Read the model definition and answer for the solid it produces. Units are mm, in the model's axes. Face numbers are marked on the shaded views. Coordinates: 2 decimals unless noted, no trailing zeros. Loops run counter-clockwise (first coordinate to the right, second up) from the corner with the lowest first, then second, coordinate; pieces in that order, holes last. Notation, with made-up numbers: (68.5, -24.5) - (102.5, -24.5) arc R11 cw to (102.5, -14.5) - close; hole circle Ø11 at (71.25, 69.25). An arc over 180 degrees is marked (long way). Use one line per item in the form item = value. Start each with the question number.
1) A cutting plane is placed at D-D (z = -13.5). Give the vertices of the cut face in (x, y), and give its area (3 significant figures).
2) The mould has two halves that part along Z. Classify the marked faces 1, 2 and 3: released by +Z, released by -Z, zero draft, split by the parting line, or undercut.
3) A cutting plane is placed at A-A (z = 6). Give the vertices of the cut face in (x, y) (3 decimals).
4) A cutting plane is placed at C-C (x = -11). Give the vertices of the cut face in (y, z).
5) Consider line 1 (Z direction, x = 22, y = 3.6); line 2 (X direction, y = 3.45, z = 14.5); line 3 (X direction, y = 0.85, z = -10). Determine where each line is inside the solid, lowest interval first.
6) This flat-tipped pin is pushed along its axis until it touches: P1, Ø2, axis at x = 21, z = 14.5, coming from the +Y side. Where does it stop, or does it pass through?
7) A cutting plane is placed at B-B (y = 4.3). Give the vertices of the cut face in (x, z).
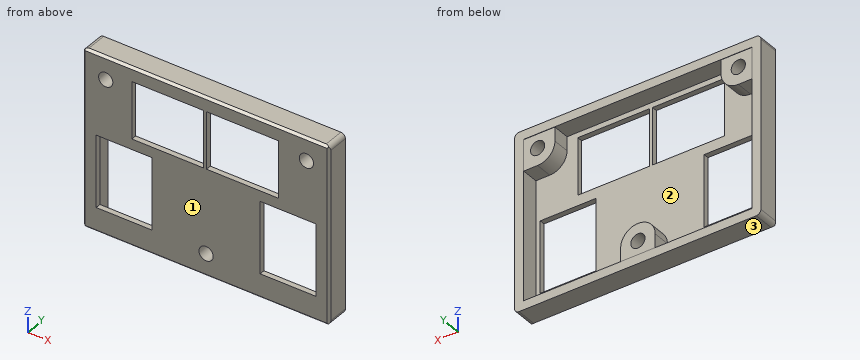
from build123d import *

# Parameters (mm, degrees)
SKETCH1_W           = 54
SKETCH1_H           = 39
BOSS_EXTRUDE1_DEPTH = 5
SKETCH2_W           = 50.1
SKETCH2_H           = 35.1
CUT_EXTRUDE1_DEPTH  = 0.0762
CUT_EXTRUDE2_DEPTH  = 3.75
SKETCH4_R           = 1.56
CUT_EXTRUDE3_DEPTH  = 34.667399758
SKETCH6_W           = 12.25
SKETCH6_H           = 15.75
SKETCH6_W_2         = 15.75
SKETCH6_H_2         = 12.5
CUT_EXTRUDE5_DEPTH  = 34.524465789
CHAMFER1_SIZE       = 0.5
FILLET1_R           = 1


with BuildPart() as part:
    # Sketch1 → Boss-Extrude1 (new body)
    with BuildSketch(Plane(origin=(0, 0, 0), x_dir=(1, 0, 0), z_dir=(0, 1, 0))):
        Rectangle(SKETCH1_W, SKETCH1_H)
    extrude(amount=BOSS_EXTRUDE1_DEPTH)

    # Sketch2 → Cut-Extrude1 (cut)
    with BuildSketch(Plane(origin=(0, 5, 0), x_dir=(1, 0, 0), z_dir=(0, 1, 0))):
        Rectangle(SKETCH2_W, SKETCH2_H)
    extrude(amount=-CUT_EXTRUDE1_DEPTH, mode=Mode.SUBTRACT)

    # Sketch3 → Cut-Extrude2 (cut)
    with BuildSketch(Plane(origin=(0, 4.9238, 0), x_dir=(1, 0, 0), z_dir=(0, 1, 0))):
        with BuildLine():
            Line((-3.79, 14.5), (-3.79, 17.55))
            Line((-3.79, 17.55), (-25.05, 17.55))
            Line((-25.05, 17.55), (-25.05, -10.71))
            Line((-25.05, -10.71), (-22, -10.71))
            ThreePointArc((-22, -10.71), (-19.320065299, -11.820065299), (-18.21, -14.5))
            Line((-18.21, -14.5), (-18.21, -17.55))
            Line((-18.21, -17.55), (18.21, -17.55))
            Line((18.21, -17.55), (18.21, -14.5))
            ThreePointArc((18.21, -14.5), (19.320065299, -11.820065299), (22, -10.71))
            Line((22, -10.71), (25.05, -10.71))
            Line((25.05, -10.71), (25.05, 17.55))
            Line((25.05, 17.55), (3.79, 17.55))
            Line((3.79, 17.55), (3.79, 14.5))
            ThreePointArc((3.79, 14.5), (0, 10.71), (-3.79, 14.5))
        make_face()
    extrude(amount=-CUT_EXTRUDE2_DEPTH, mode=Mode.SUBTRACT)

    # Sketch4 → Cut-Extrude3 (cut, through all)
    with BuildSketch(Plane(origin=(0, 4.9238, 0), x_dir=(1, 0, 0), z_dir=(0, 1, 0))):
        with Locations(Location((0, 14.5, 0), (0, 0, 270))):
            Circle(SKETCH4_R)
        with Locations(Location((-22, -14.5, 0), (0, 0, 270))):
            Circle(SKETCH4_R)
        with Locations(Location((22, -14.5, 0), (0, 0, 90))):
            Circle(SKETCH4_R)
    extrude(amount=-CUT_EXTRUDE3_DEPTH, mode=Mode.SUBTRACT)

    # Sketch6 → Cut-Extrude5 (cut, through all)
    with BuildSketch(Plane(origin=(0, 1.1738, 0), x_dir=(1, 0, 0), z_dir=(0, 1, 0))):
        with Locations((17.975, 6.255)):
            Rectangle(SKETCH6_W, SKETCH6_H)
        with Locations((7.975, -10.15)):
            Rectangle(SKETCH6_W_2, SKETCH6_H_2)
        with Locations((-17.975, 6.255)):
            Rectangle(SKETCH6_W, SKETCH6_H)
        with Locations((-8.4, -10.15)):
            Rectangle(SKETCH6_W_2, SKETCH6_H_2)
    extrude(amount=-CUT_EXTRUDE5_DEPTH, mode=Mode.SUBTRACT)

    # Chamfer1
    chamfer1_edges = [part.edges().sort_by_distance(p)[0] for p in [
        (-27, 0, 0),
        (0, 0, -19.5),
        (27, 0, 0),
        (0, 0, 19.5),
    ]]
    chamfer(chamfer1_edges, length=CHAMFER1_SIZE)

    # Fillet1
    fillet1_edges = [part.edges().sort_by_distance(p)[0] for p in [
        (-27, 2.75, 19.5),
        (-27, 2.75, -19.5),
        (27, 2.75, -19.5),
        (27, 2.75, 19.5),
    ]]
    fillet(fillet1_edges, radius=FILLET1_R)


solid = part.part
Found:
q1.outline = (-27, 0.5) - (-26.5, 0) - (-24.1, 0) - (-24.1, 1.17) - (-25.05, 1.17) - (-25.05, 5) - (-27, 5) - close; (-11.85, 0) - (-1.2, 0) - (-1.2, 4.92) - (-3.66, 4.92) - (-3.66, 1.17) - (-11.85, 1.17) - close; (1.2, 0) - (11.85, 0) - (11.85, 1.17) - (3.66, 1.17) - (3.66, 4.92) - (1.2, 4.92) - close; (24.1, 0) - (26.5, 0) - (27, 0.5) - (27, 5) - (25.05, 5) - (25.05, 1.17) - (24.1, 1.17) - close
q1.area = 64.9 mm^2
q2.face_1 = zero draft
q2.face_2 = undercut
q2.face_3 = released by -Z
q3.outline = (-27, 0.5) - (-26.5, 0) - (-16.275, 0) - (-16.275, 1.174) - (-25.05, 1.174) - (-25.05, 5) - (-27, 5) - close; (-0.525, 0) - (0.1, 0) - (0.1, 1.174) - (-0.525, 1.174) - close; (15.85, 0) - (26.5, 0) - (27, 0.5) - (27, 5) - (25.05, 5) - (25.05, 1.174) - (15.85, 1.174) - close
q4.outline = (0, -19) - (0.5, -19.5) - (5, -19.5) - (5, -17.55) - (1.17, -17.55) - (1.17, 3.9) - (0, 3.9) - close; (0, 16.4) - (1.17, 16.4) - (1.17, 17.55) - (5, 17.55) - (5, 19.5) - (0.5, 19.5) - (0, 19) - close
q5.line_1 = -19.5 to -17.55, 10.71 to 12.94, 16.06 to 19.5
q5.line_2 = -27 to -23.56, -20.44 to -18.21, 18.21 to 20.44, 23.56 to 27
q5.line_3 = -27 to -24.1, -11.85 to 11.85, 24.1 to 27
q6.P1 = 4.92
q7.outline = (-27, -18.5) arc R1 ccw to (-26, -19.5) - (26, -19.5) arc R1 ccw to (27, -18.5) - (27, 18.5) arc R1 ccw to (26, 19.5) - (-26, 19.5) arc R1 ccw to (-27, 18.5) - close; hole (-25.05, -17.55) - (-3.79, -17.55) - (-3.79, -14.5) arc R3.79 cw to (3.79, -14.5) - (3.79, -17.55) - (25.05, -17.55) - (25.05, 10.71) - (22, 10.71) arc R3.79 cw to (18.21, 14.5) - (18.21, 17.55) - (-18.21, 17.55) - (-18.21, 14.5) arc R3.79 cw to (-22, 10.71) - (-25.05, 10.71) - close; hole circle Ø3.12 at (-22, 14.5); hole circle Ø3.12 at (0, -14.5); hole circle Ø3.12 at (22, 14.5)
